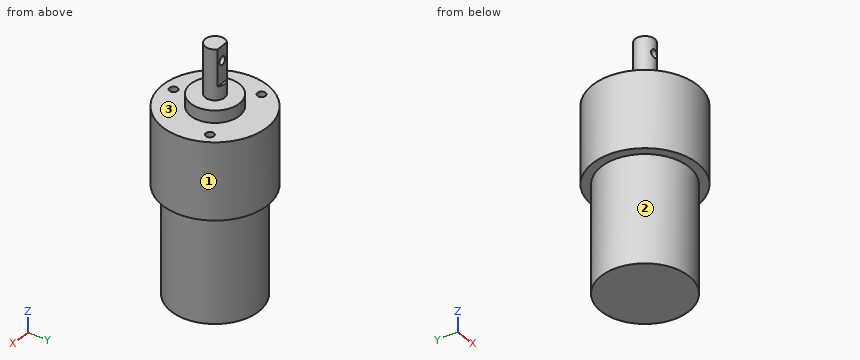
```python
from build123d import *

# Parameters (mm, degrees)
SKETCH_1_R          = 21.5
SKETCH_1_R_2        = 18
EXTRUDE_1_DEPTH     = 31.5
SKETCH_1_3_R        = 18
EXTRUDE_2_DEPTH     = 44
SKETCH_2_R          = 10
SKETCH_2_R_2        = 4
EXTRUDE_3_DEPTH     = 5
SKETCH_2_2_R        = 4
EXTRUDE_4_DEPTH     = 25.5
CUT_EXTRUDE_START   = 3
SKETCH_3_W          = 15.90617044
SKETCH_3_H          = 15
CUT_EXTRUDE_1_DEPTH = 62.602631525
M4X0_7_1_D          = 3.3
M4X0_7_1_DEPTH      = 11.5
M4X0_7_1_TIP        = 0.991420021
M4X0_7_2_D          = 3.3


with BuildPart() as part:
    # ｽｹｯﾁ1 → ﾎﾞｽ - 押し出し1 (new body)
    with BuildSketch(Plane.XY):
        Circle(SKETCH_1_R)
        Circle(SKETCH_1_R_2, mode=Mode.SUBTRACT)
        Circle(SKETCH_1_R_2)
    extrude(amount=EXTRUDE_1_DEPTH)

    # ｽｹｯﾁ1<3> → ﾎﾞｽ - 押し出し2 (add)
    with BuildSketch(Plane.XY):
        Circle(SKETCH_1_3_R)
    extrude(amount=-EXTRUDE_2_DEPTH)

    # ｽｹｯﾁ2 → ﾎﾞｽ - 押し出し3 (add)
    with BuildSketch(Plane.XY.offset(31.5)):
        Circle(SKETCH_2_R)
        Circle(SKETCH_2_R_2, mode=Mode.SUBTRACT)
    extrude(amount=EXTRUDE_3_DEPTH)

    # ｽｹｯﾁ2<2> → ﾎﾞｽ - 押し出し4 (add)
    with BuildSketch(Plane.XY.offset(31.5)):
        Circle(SKETCH_2_2_R)
    extrude(amount=EXTRUDE_4_DEPTH)

    # ｽｹｯﾁ3 → ｶｯﾄ - 押し出し1 (cut, through all)
    with BuildSketch(Plane(origin=(0, 0, 0), x_dir=(1, 0, 0), z_dir=(0, 1, 0)).offset(CUT_EXTRUDE_START)):
        with Locations((0, -49.5)):
            Rectangle(SKETCH_3_W, SKETCH_3_H)
    extrude(amount=CUT_EXTRUDE_1_DEPTH, mode=Mode.SUBTRACT)

    # M4x0.7 ねじ穴1
    with Locations(Plane.XY.offset(31.5)):
        with Locations((0, -17), (-14.722431864, 8.5), (14.722431864, 8.5)):
            Hole(M4X0_7_1_D / 2, depth=M4X0_7_1_DEPTH)
            with Locations((0, 0, -(M4X0_7_1_DEPTH + M4X0_7_1_TIP / 2))):  # 118° drill point
                Cone(0, M4X0_7_1_D / 2, M4X0_7_1_TIP, mode=Mode.SUBTRACT)

    # M4x0.7 ねじ穴2 (through all)
    with Locations(Plane(origin=(0, 3, 0), x_dir=(1, 0, 0), z_dir=(0, 1, 0))):
        with Locations((0, -51)):
            Hole(M4X0_7_2_D / 2)


solid = part.part
```
The model under review builds one solid part; all positions refer to its coordinate system, in mm. Face numbers are marked on the shaded views. A direction names the side the tool comes from. Give positions to 0.01 mm unless a question says otherwise; leave off trailing zeros. Write each loop counter-clockwise with the first axis right and the second up, starting at its lowest first coordinate (ties: lowest second). Pieces come first, ordered by that corner, then holes. Notation, with made-up numbers: (-0.5, 26) -> (4.5, 26) arc R12 ccw to (4.5, 48) -> close; hole circle Ø3 at (4.25, 64). An arc over 180 degrees is marked (long way). Put each result on its own line as item: value.
(1) Tool access review of the marked faces 1, 2 and 3: name each direction out of +Z, -Z, +X, -X, +Y, -Y from which nothing blocks a thin tool from reaching the whole face with its end or side.
Results are:
face 1: +Z, -Z
face 2: -Z
face 3: +Z
(2) To check wall thickness, follow probe 1 along Z at (x, y) = (0, -1); probe 2 along X at (y, z) = (8.5, 23); probe 3 along X at (y, z) = (10, 21.5). State the ranges of each line that lie inside material, in increasing order. Write a range as from..to.
Results are:
probe 1: -44..49.35, 52.65..57
probe 2: -19.75..-16.37, -13.07..13.07, 16.37..19.75
probe 3: -19.03..-15.41, -14.04..14.04, 15.41..19.03
(3) We need section B-B, the plane z = 51. Give the boundary of the cut face in (x, y), and give its area (3 significant figures).
Results are:
outline: (-2.65, 3) arc R4 ccw to (-1.65, -3.64) -> (-1.65, 3) -> close; (1.65, -3.64) arc R4 ccw to (2.65, 3) -> (1.65, 3) -> close
area: 23.9 mm²
(4) For pin 1 Ø2 at (y, z) = (-6.5, -7) entering from -X; pin 2 Ø2.5 at (x, z) = (0.5, 49.5) entering from +Y; pin 3 Ø0.5 at (x, y) = (-1, 3.5) entering from +Z, all flat-tipped, find the tip position at first contact; note any pin that passes through.
Results are:
pin 1: x = -17.14
pin 2: y = 3
pin 3: z = 42
(5) We need section A-A, the plane y = 0. Give the boundary of the cut face in (x, z), and give its area (3 significant figures).
Results are:
outline: (-21.5, 0) -> (-18, 0) -> (-18, -44) -> (18, -44) -> (18, 0) -> (21.5, 0) -> (21.5, 31.5) -> (10, 31.5) -> (10, 36.5) -> (4, 36.5) -> (4, 57) -> (-4, 57) -> (-4, 36.5) -> (-10, 36.5) -> (-10, 31.5) -> (-21.5, 31.5) -> close; hole circle Ø3.3 at (0, 51)
area: 3,190 mm²
(6) We need section D-D, the plane z = -25. Give the boundary of the cut face in (x, y).
Results are:
outline: circle Ø36 at (0, 0)
(7) We need section C-C, the plane y = -8. Give the boundary of the cut face in (x, z), and give its area (3 significant figures).
Results are:
outline: (-19.96, 0) -> (-16.12, 0) -> (-16.12, -44) -> (16.12, -44) -> (16.12, 0) -> (19.96, 0) -> (19.96, 31.5) -> (6, 31.5) -> (6, 36.5) -> (-6, 36.5) -> (-6, 31.5) -> (-19.96, 31.5) -> close
area: 2,740 mm²
